Source: CAD feature listing. Evaluate the final solid. Frame: model axes, mm. A direction names the side the tool comes from. Coordinates: 2 decimals unless noted, no trailing zeros. Loops run counter-clockwise (first coordinate to the right, second up) from the corner with the lowest first, then second, coordinate; pieces in that order, holes last.
from build123d import *

# Parameters (mm, degrees)
BODY_DEPTH   = 8.9
TOPCUTSKE_W  = 8.89
TOPCUTSKE_H  = 8.89
TOPCUT_DEPTH = 8.9


with BuildPart() as part:
    # BodySke → Body (new body)
    with BuildSketch(Plane(origin=(0, 0, 0), x_dir=(0, 0, -1), z_dir=(1, 0, 0))):
        with BuildLine():
            Line((-5.715, -9), (5.715, -9))
            Line((5.715, -9), (5.715, -8.4))
            Line((5.715, -8.4), (4.695, -8.4))
            Line((4.695, -8.4), (4.695, -8.1))
            Line((4.695, -8.1), (4.95, -8.1))
            Line((4.95, -8.1), (4.95, -7.5))
            Line((4.95, -7.5), (4.338530006, -5.82))
            Line((4.338530006, -5.82), (3.223696854, -5.82))
            ThreePointArc((3.223696854, -5.82), (2.08483996, -4.983958225), (2.54124896, -3.646927299))
            ThreePointArc((2.54124896, -3.646927299), (4.44393925, 0.097102731), (2.379524457, 3.754449142))
            Line((2.379524457, 3.754449142), (0.985, 1.554147676))
            ThreePointArc((0.985, 1.554147676), (0, -1.84), (-0.985, 1.554147676))
            Line((-0.985, 1.554147676), (-2.379524457, 3.754449142))
            ThreePointArc((-2.379524457, 3.754449142), (-4.44393925, 0.097102731), (-2.54124896, -3.646927299))
            ThreePointArc((-2.54124896, -3.646927299), (-2.08483996, -4.983958225), (-3.223696854, -5.82))
            Line((-3.223696854, -5.82), (-4.338530006, -5.82))
            Line((-4.338530006, -5.82), (-4.95, -7.5))
            Line((-4.95, -7.5), (-4.95, -8.1))
            Line((-4.95, -8.1), (-4.695, -8.1))
            Line((-4.695, -8.1), (-4.695, -8.4))
            Line((-4.695, -8.4), (-5.715, -8.4))
            Line((-5.715, -8.4), (-5.715, -9))
        make_face()
    extrude(amount=BODY_DEPTH)

    # TopCutSke → TopCut (cut)
    with BuildSketch(Plane.ZY):
        with Locations((0, 7.5565)):
            Rectangle(TOPCUTSKE_W, TOPCUTSKE_H)
    extrude(amount=-TOPCUT_DEPTH, mode=Mode.SUBTRACT)


solid = part.part
Q1. Section A-A, the plane y = 0. Return the cut outline in (x, z) (3 decimals).
Q2. Draft query along Z for faces 1 (the cylindrical face through (4.39, -0.47, -4.42)), 2 (the flat face through (4, 3.111, 3)), 3 (the flat face through (4.39, -6.65, 4.64)), 4 (the cylindrical face through (4.39, -1.84, -0.07)). Return one class per face: +Z half, -Z half, draft (parallel to the pull), parting line (faces both ways), or undercut.
Q3. Section B-B, the plane z = -2.75. Return the cut outline in (x, y), plus the area to 3 significant figures.
Q4. Access query for faces 5 (the flat face through (4, -8.4, -5)), 6 (the flat face through (0, -4, 0)), 7 (the flat face through (4, -5.82, 4)), 8 (the flat face through (4.388, 2.344, -1.485)). Directions: +Z, -Z, +X, -X, +Y, -Y. A direction counts if a zero-diameter tool reaches every point of the face in a straight line with its end or side. Return the directions, or none.
Q5. Contact query for flat-ended pins moving along their axis: pin 1 Ø1.2 at (x, z) = (5, 4) entering from +Y; pin 2 Ø5 at (y, z) = (0, 0) entering from +X; pin 3 Ø1.5 at (x, y) = (3, -3.5) entering from -Z; pin 4 Ø1 at (x, y) = (2, -4.5) entering from +Z. Output: stop coordinate, or through.
Q6. Line query: line 1 along Z through (x, y) = (5.5, 0) (3 decimals); line 2 along Y through (x, z) = (4.5, 0); line 3 along Y through (x, z) = (7, -3). Output: solid intervals per line, ascending.
Q7. Section D-D, the plane z = 0. Return the cut outline in (x, y).
Derived:
1. outline: (0, -4.445) - (8.9, -4.445) - (8.9, -1.84) - (0, -1.84) - close; (0, 1.84) - (8.9, 1.84) - (8.9, 4.445) - (0, 4.445) - close
2. face 1: -Z half
2. face 2: draft
2. face 3: +Z half
2. face 4: undercut
3. outline: (0, -9) - (8.9, -9) - (8.9, -5.72) - (0, -5.72) - close; (0, -3.49) - (8.9, -3.49) - (8.9, 3.11) - (0, 3.11) - close
3. area: 87.9 mm2
4. face 5: -Z, +X, -X
4. face 6: +Z, -Z, -X, +Y, -Y
4. face 7: +Z, +X, -X
4. face 8: +X, -X, +Y
5. pin 1: stops at y = 2.86
5. pin 2: stops at x = 8.9
5. pin 3: stops at z = -3.49
5. pin 4: stops at z = 2.21
6. line 1: z = -4.445 to -1.84, 1.84 to 4.445
6. line 2: y = -9 to -1.84
6. line 3: y = -9 to -5.8, -3.28 to 3.11
7. outline: (0, -9) - (8.9, -9) - (8.9, -1.84) - (0, -1.84) - close
